from build123d import *

# Parameters (mm, degrees)
SKETCH1_W           = 141.761639
SKETCH1_H           = 75.858415486
BOSS_EXTRUDE1_DEPTH = 3.175
SKETCH2_R           = 3.5625
CUT_EXTRUDE1_DEPTH  = 10
SKETCH3_W           = 72
SKETCH3_H           = 25
CUT_EXTRUDE2_DEPTH  = 10
SKETCH4_R           = 1.5
CUT_EXTRUDE3_DEPTH  = 10
SKETCH5_R           = 1.5
CUT_EXTRUDE4_DEPTH  = 10
SKETCH7_W           = 4
SKETCH7_H           = 2.5
SKETCH7_H_2         = 3
CUT_EXTRUDE5_DEPTH  = 10


with BuildPart() as part:
    # Sketch1 → Boss-Extrude1 (new body)
    with BuildSketch(Plane(origin=(0, 0, 0), x_dir=(1, 0, 0), z_dir=(0, 1, 0))):
        Rectangle(SKETCH1_W, SKETCH1_H)
    extrude(amount=BOSS_EXTRUDE1_DEPTH)

    # Sketch2 → Cut-Extrude1 (cut)
    with BuildSketch(Plane(origin=(0, 3.175, 0), x_dir=(1, 0, 0), z_dir=(0, 1, 0))):
        with Locations(Location((-35.4408195, -17.929207743, 0), (0, 0, 270))):
            Circle(SKETCH2_R)
        with Locations(Location((0, -17.929207743, 0), (0, 0, 270))):
            Circle(SKETCH2_R)
        with Locations(Location((35.4408195, -17.929207743, 0), (0, 0, 270))):
            Circle(SKETCH2_R)
    extrude(amount=-CUT_EXTRUDE1_DEPTH, mode=Mode.SUBTRACT)

    # Sketch3 → Cut-Extrude2 (cut)
    with BuildSketch(Plane(origin=(0, 3.175, 0), x_dir=(1, 0, 0), z_dir=(0, 1, 0))):
        with Locations((0, 9.485)):
            Rectangle(SKETCH3_W, SKETCH3_H)
    extrude(amount=-CUT_EXTRUDE2_DEPTH, mode=Mode.SUBTRACT)

    # Sketch4 → Cut-Extrude3 (cut)
    with BuildSketch(Plane(origin=(0, 3.175, 0), x_dir=(1, 0, 0), z_dir=(0, 1, 0))):
        with Locations(Location((37.7, 25.485, 0), (0, 0, 270))):
            Circle(SKETCH4_R)
        with Locations(Location((37.7, -5.515, 0), (0, 0, 270))):
            Circle(SKETCH4_R)
        with Locations(Location((-37.3, -5.515, 0), (0, 0, 270))):
            Circle(SKETCH4_R)
        with Locations(Location((-37.3, 25.485, 0), (0, 0, 270))):
            Circle(SKETCH4_R)
    extrude(amount=-CUT_EXTRUDE3_DEPTH, mode=Mode.SUBTRACT)

    # Sketch5 → Cut-Extrude4 (cut)
    with BuildSketch(Plane(origin=(0, 3.175, 0), x_dir=(1, 0, 0), z_dir=(0, 1, 0))):
        with Locations(Location((68.8808195, 0, 0), (0, 0, 270))):
            Circle(SKETCH5_R)
        with Locations(Location((-68.8808195, 0, 0), (0, 0, 270))):
            Circle(SKETCH5_R)
    extrude(amount=-CUT_EXTRUDE4_DEPTH, mode=Mode.SUBTRACT)

    # Sketch7 → Cut-Extrude5 (cut)
    with BuildSketch(Plane.XZ):
        with Locations((-35.4408195, 9.975414813)):
            Rectangle(SKETCH7_W, SKETCH7_H)
        Polygon((9.399912783, 19.969203639), (6.40097942, 19.889211847), (6.453259422, 17.929207743), (6.40097942, 15.969203639), (9.399912783, 15.889211847), (9.454326439, 17.929207743), align=None)
        with Locations((35.4408195, 25.849658905)):
            Rectangle(SKETCH7_W, SKETCH7_H_2)
    extrude(amount=-CUT_EXTRUDE5_DEPTH, mode=Mode.SUBTRACT)


solid = part.part
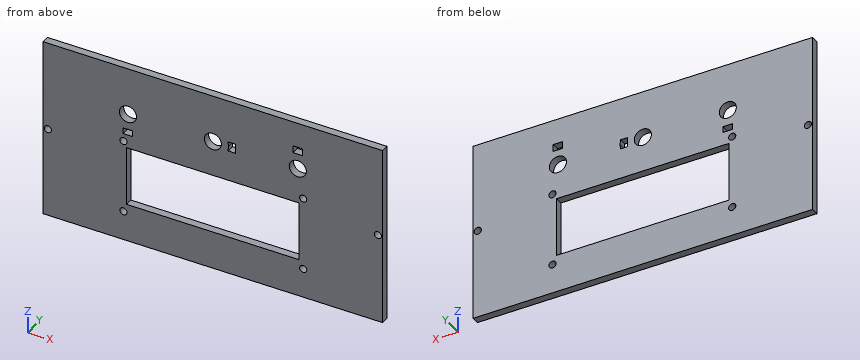
The listing builds one solid part. Answer for the finished solid, in the listing's coordinates (mm). Coordinates: 2 decimals unless noted, no trailing zeros. Write each loop counter-clockwise with the first axis right and the second up, starting at its lowest first coordinate (ties: lowest second). Pieces come first, ordered by that corner, then holes. Notation, with made-up numbers: M -2,-3 L 3,-3 A9 cw 3,14 Z; hole C 17.5,65 d5. An arc over 180 degrees is marked long. Use one line per item in the form item = value.
Item 1: Find section C-C, the plane z = -10. Give the vertices of the cut face in (x, y) (3 decimals).
Model answer:
outline = M -70.881,0 L -36,0 L -36,3.175 L -70.881,3.175 Z; M 36,0 L 70.881,0 L 70.881,3.175 L 36,3.175 Z
Item 2: Find section A-A, the plane z = 0. Give the vertices of the cut face in (x, y) (3 decimals).
Model answer:
outline = M -70.881,0 L -70.381,0 L -70.381,3.175 L -70.881,3.175 Z; M -67.381,0 L -36,0 L -36,3.175 L -67.381,3.175 Z; M 36,0 L 67.381,0 L 67.381,3.175 L 36,3.175 Z; M 70.381,0 L 70.881,0 L 70.881,3.175 L 70.381,3.175 Z
Item 3: Find section B-B, the plane x = 19. Give the vertices of the cut face in (y, z) (3 decimals).
Model answer:
outline = M 0,-37.929 L 3.175,-37.929 L 3.175,-21.985 L 0,-21.985 Z; M 0,3.015 L 3.175,3.015 L 3.175,37.929 L 0,37.929 Z
Item 4: Find the intervals of material crossed by probe 1 along X at (y, z) = (2.2, 0); probe 2 along X at (y, z) = (2.2, 25); probe 3 along Z at (x, y) = (-6.5, 1.05) (3 decimals), in increasing order.
Model answer:
probe_1 = -70.88 to -70.38, -67.38 to -36, 36 to 67.38, 70.38 to 70.88
probe_2 = -70.88 to 33.44, 37.44 to 70.88
probe_3 = -37.929 to -21.985, 3.015 to 37.929
Item 5: Find section D-D, the plane x = 0. Give the vertices of the cut face in (y, z) (3 decimals).
Model answer:
outline = M 0,-37.929 L 3.175,-37.929 L 3.175,-21.985 L 0,-21.985 Z; M 0,3.015 L 3.175,3.015 L 3.175,14.367 L 0,14.367 Z; M 0,21.492 L 3.175,21.492 L 3.175,37.929 L 0,37.929 Z
